Autodesk Fusion 360 part; units mm, degrees
sketch "スケッチ1" plane through (0, 0, 0) normal (0, 0, 1) x (1, 0, 0)
  line L0 (-1.75, -4.25) -> (1.75, -4.25)
  line L1 (1.75, -4.25) -> (1.75, 4.25)
  line L2 (1.75, 4.25) -> (-1.75, 4.25)
  line L3 (-1.75, 4.25) -> (-1.75, -4.25)
  line L4 (0, 1.75) -> (0, 22.5)
  line L5 (1.75, 0) -> (22.5, 0)
  circle A0 centre (0, 0) radius 0.25
  dimension "d1" = 3.5
  dimension "d2" = 8.5
  dimension "d9" = 0.5
extrude "押し出し1" add sketch "スケッチ1" along normal blind 3.6 contours L0 L1 L2 L3 | A0
sketch "スケッチ2" plane through (0, 0, 3.6) normal (0, 0, 1) x (-1, 0, 0)
  line L0 (1.75, -4.25) -> (1.75, 4.25)
  line L1 (1.75, 4.25) -> (-1.75, 4.25)
  line L2 (-1.75, 4.25) -> (-1.75, -4.25)
  line L3 (-1.75, -4.25) -> (1.75, -4.25)
  line L4 (0.75, -1.75) -> (-0.75, -1.75)
  line L5 (-0.75, -1.75) -> (-0.75, -0.25)
  line L6 (-0.75, -0.25) -> (0.75, -0.25)
  line L7 (0.75, -0.25) -> (0.75, -1.75)
  line L8 (-1.75, 0) -> (-22.5, 0)
  line L9 (0, -1.75) -> (0, -22.5)
  dimension "d5" = 1.5
  dimension "d6" = 1.5
  dimension "d16" = 1.75
extrude "押し出し2" add sketch "スケッチ2" along normal blind 3 contours L4 L5 L6 L7
extrude "押し出し3" add sketch "スケッチ1" against normal blind 3 contours A0
pattern_linear "R パターン1" count 3 spacing 1.27 along (0, -1, 0) both ways of "押し出し3"
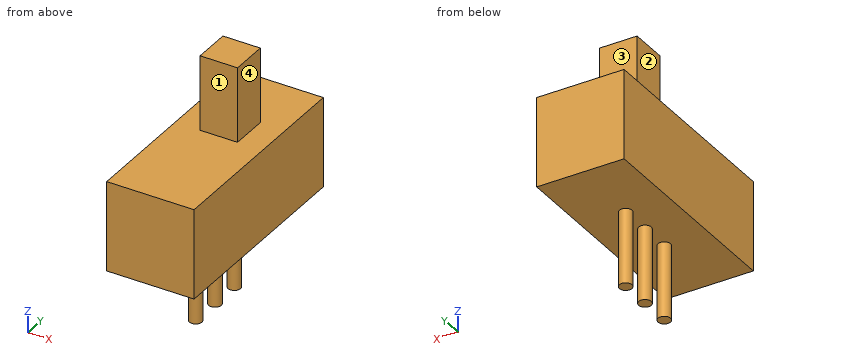
Verification items for the finished model (mm, model axes). Face numbers are marked on the shaded views. A direction names the side the tool comes from. Give positions to 0.01 mm unless a question says otherwise; leave off trailing zeros. Loops run counter-clockwise (first coordinate to the right, second up) from the corner with the lowest first, then second, coordinate; pieces in that order, holes last.
1. Section check D-D, the plane y = 1.27. Enter the section's corners in (x, z).
2. Section check B-B, the plane z = -2.25. Enter the section's corners in (x, y), then the cut area to 3 significant figures.
3. Set-up check for the marked faces 1, 2, 3 and 4: record each of +Z, -Z, +X, -X, +Y, -Y from which the full face is reachable in a straight line by a thin tool's end or side.
4. Section check A-A, the plane y = -1.27. Enter the section's corners in (x, z), then the cut area to 3 significant figures.
5. Go/stop test with flat-tipped pins: pin 1 Ø1.6 at (y, z) = (1, 5.5) entering from +X; pin 2 Ø1.8 at (x, y) = (-0.5, -0.5) entering from -Z; pin 3 Ø0.8 at (y, z) = (1, 6) entering from -X; pin 4 Ø0.8 at (x, z) = (0, 4.5) entering from -Y. Record where each tip stops, or that it passes through.
6. Section check C-C, the plane x = 0. Enter the section's corners in (y, z).
7. Thickness scan on line 1 (Z direction, x = -1.35, y = -0.25). Record the ranges inside material, lowest first.
Geometry says:
1. outline: (-1.75, 0) - (-0.25, 0) - (-0.25, -3) - (0.25, -3) - (0.25, 0) - (1.75, 0) - (1.75, 3.6) - (0.75, 3.6) - (0.75, 6.6) - (-0.75, 6.6) - (-0.75, 3.6) - (-1.75, 3.6) - close
2. outline: circle Ø0.5 at (0, -1.27); circle Ø0.5 at (0, 0); circle Ø0.5 at (0, 1.27)
2. area: 0.589 mm2
3. face 1: +Z, +X, -X, -Y
3. face 2: +Z, -X, +Y, -Y
3. face 3: +Z, +X, -X, +Y
3. face 4: +Z, +X, +Y, -Y
4. outline: (-1.75, 0) - (-0.25, 0) - (-0.25, -3) - (0.25, -3) - (0.25, 0) - (1.75, 0) - (1.75, 3.6) - (-1.75, 3.6) - close
4. area: 14.1 mm2
5. pin 1: stops at x = 0.75
5. pin 2: stops at z = -3
5. pin 3: stops at x = -0.75
5. pin 4: stops at y = 0.25
6. outline: (-4.25, 0) - (-1.52, 0) - (-1.52, -3) - (-1.02, -3) - (-1.02, 0) - (-0.25, 0) - (-0.25, -3) - (0.25, -3) - (0.25, 0) - (1.02, 0) - (1.02, -3) - (1.52, -3) - (1.52, 0) - (4.25, 0) - (4.25, 3.6) - (1.75, 3.6) - (1.75, 6.6) - (0.25, 6.6) - (0.25, 3.6) - (-4.25, 3.6) - close
7. line 1: z = 0 to 3.6
